Here's how the part is built. I have some questions about the finished solid (model axes, mm). Give positions to 0.01 mm unless a question says otherwise; leave off trailing zeros. Write each loop counter-clockwise with the first axis right and the second up, starting at its lowest first coordinate (ties: lowest second). Pieces come first, ordered by that corner, then holes. Notation, with made-up numbers: (82, 38) - (103, 38) arc R20 ccw to (103, 46) - close; hole circle Ø11 at (23.5, 40). An arc over 180 degrees is marked (long way). Use a Markdown table: item, result.
```python
from build123d import *

# Parameters (mm, degrees)
SKETCH4_W           = 203.2
SKETCH4_H           = 203.2
SKETCH4_R           = 6.35
SKETCH4_R_2         = 32.004
BOSS_EXTRUDE1_DEPTH = 4.7625


with BuildPart() as part:
    # Sketch4 → Boss-Extrude1 (new body)
    with BuildSketch(Plane.XY):
        Rectangle(SKETCH4_W, SKETCH4_H)
        with Locations((-54.018973032, 17.551828308)):
            Circle(SKETCH4_R, mode=Mode.SUBTRACT)
        with Locations((0, 56.798909535)):
            Circle(SKETCH4_R, mode=Mode.SUBTRACT)
        with Locations((-33.385561371, -45.951283076)):
            Circle(SKETCH4_R, mode=Mode.SUBTRACT)
        with Locations((33.385561371, -45.951283076)):
            Circle(SKETCH4_R, mode=Mode.SUBTRACT)
        with Locations((54.018973032, 17.551828308)):
            Circle(SKETCH4_R, mode=Mode.SUBTRACT)
        Circle(SKETCH4_R_2, mode=Mode.SUBTRACT)
    extrude(amount=BOSS_EXTRUDE1_DEPTH)


solid = part.part
```
Item 1: If we section it at A-A, the plane x = 0: Write out the boundary of the cut face in (y, z), plus the area to 3 significant figures.
Values:
| item | result |
|---|---|
| outline | (-101.6, 0) - (-32, 0) - (-32, 4.76) - (-101.6, 4.76) - close; (32, 0) - (50.45, 0) - (50.45, 4.76) - (32, 4.76) - close; (63.15, 0) - (101.6, 0) - (101.6, 4.76) - (63.15, 4.76) - close |
| area | 602 mm2 |
Item 2: If we section it at B-B, the plane y = 28.5: Write out the boundary of the cut face in (x, z).
Values:
| item | result |
|---|---|
| outline | (-101.6, 0) - (-14.56, 0) - (-14.56, 4.76) - (-101.6, 4.76) - close; (14.56, 0) - (101.6, 0) - (101.6, 4.76) - (14.56, 4.76) - close |
Item 3: If we section it at D-D, the plane x = -22.5: Write out the boundary of the cut face in (y, z), plus the area to 3 significant figures.
Values:
| item | result |
|---|---|
| outline | (-101.6, 0) - (-22.76, 0) - (-22.76, 4.76) - (-101.6, 4.76) - close; (22.76, 0) - (101.6, 0) - (101.6, 4.76) - (22.76, 4.76) - close |
| area | 751 mm2 |
Item 4: Thinking about a two-plate mould opening in Y: for faces 1 (the flat face through (-1, -101.6, 2)), 2 (the flat face through (-24, 24, 4.762)), 3 (the cylindrical face through (-6.938, -31.243, 2.348)), 4 (the cylindrical face through (-0.8, 63.1, 2.3)), which applies, +Y half, -Y half, draft (parallel to the pull), parting line (faces both ways), or undercut?
Values:
| item | result |
|---|---|
| face 1 | -Y half |
| face 2 | draft |
| face 3 | undercut |
| face 4 | undercut |
Item 5: I need wall thicknesses on line 1 along X through (y, z) = (-46.5, 0.4); line 2 along Y through (x, z) = (0, 3.65); line 3 along X through (y, z) = (16, 3.8). Which ranges of each line are inside material? Lowest first, please. Write a range as [from, to].
Values:
| item | result |
|---|---|
| line 1 | x = [-101.6, -39.71], [-27.06, 27.06], [39.71, 101.6] |
| line 2 | y = [-101.6, -32], [32, 50.45], [63.15, 101.6] |
| line 3 | x = [-101.6, -60.18], [-47.86, -27.72], [27.72, 47.86], [60.18, 101.6] |
Item 6: Will these pins go through, and if not, where does the flat tip stop? pin 1 Ø14.5 at (x, y) = (33.39, -45.95) entering from +Z; pin 2 Ø11.5 at (x, y) = (0, 56.8) entering from -Z.
Values:
| item | result |
|---|---|
| pin 1 | stops at z = 4.76 |
| pin 2 | passes through |
Item 7: If we section it at C-C, the plane z = 3.5: Write out the boundary of the cut face in (x, y).
Values:
| item | result |
|---|---|
| outline | (-101.6, -101.6) - (101.6, -101.6) - (101.6, 101.6) - (-101.6, 101.6) - close; hole circle Ø12.7 at (-54.02, 17.55); hole circle Ø12.7 at (-33.39, -45.95); hole circle Ø64.01 at (0, 0); hole circle Ø12.7 at (0, 56.8); hole circle Ø12.7 at (33.39, -45.95); hole circle Ø12.7 at (54.02, 17.55) |
